Geometry: see drawing. Coordinates: mm, zero at the bounding-box minimum. A direction names the side the tool comes from. Coordinates: 2 decimals unless noted, no trailing zeros. Loops run counter-clockwise (first coordinate to the right, second up) from the corner with the lowest first, then second, coordinate; pieces in that order, holes last. Notation, with made-up numbers: (55, 51) -> (89, 51) arc R10 ccw to (89, 64) -> close; hole circle Ø11 at (6, -28). An arc over 180 degrees is marked (long way). One line per item, written item: value. Start each with the question number.
Item 1: Contact query for flat-ended pins moving along their axis: pin 1 Ø8 at (y, z) = (35.5, 21.5) entering from -X; pin 2 Ø1.5 at (x, z) = (17, 10) entering from +Y. Output: stop coordinate, or through.
Item 2: Ray query, probe 1 along X at (y, z) = (38, 68.5); probe 2 along Y at (x, z) = (50, 55.5). Return the intervals inside material, ascending. Write a range as from..to.
Item 3: Section query D-D on x = 21. Return loops of the section in (y, z), then the cut area to 3 significant figures.
Item 4: Section query A-A on y = 27. Return loops of the section in (x, z), then the cut area to 3 significant figures.
Item 5: Set-up query: the marked faces 1 and 2. Return all of +Z, -Z, +X, -X, +Y, -Y with unobstructed straight access to the full face (end or side cutting, diameter ignored); none if empty.
Item 6: Section query B-B on z = 39.5. Return loops of the section in (x, y), then the cut area to 3 significant figures.
Item 7: Section query C-C on z = 49.5. Return loops of the section in (x, y), then the cut area to 3 significant figures.
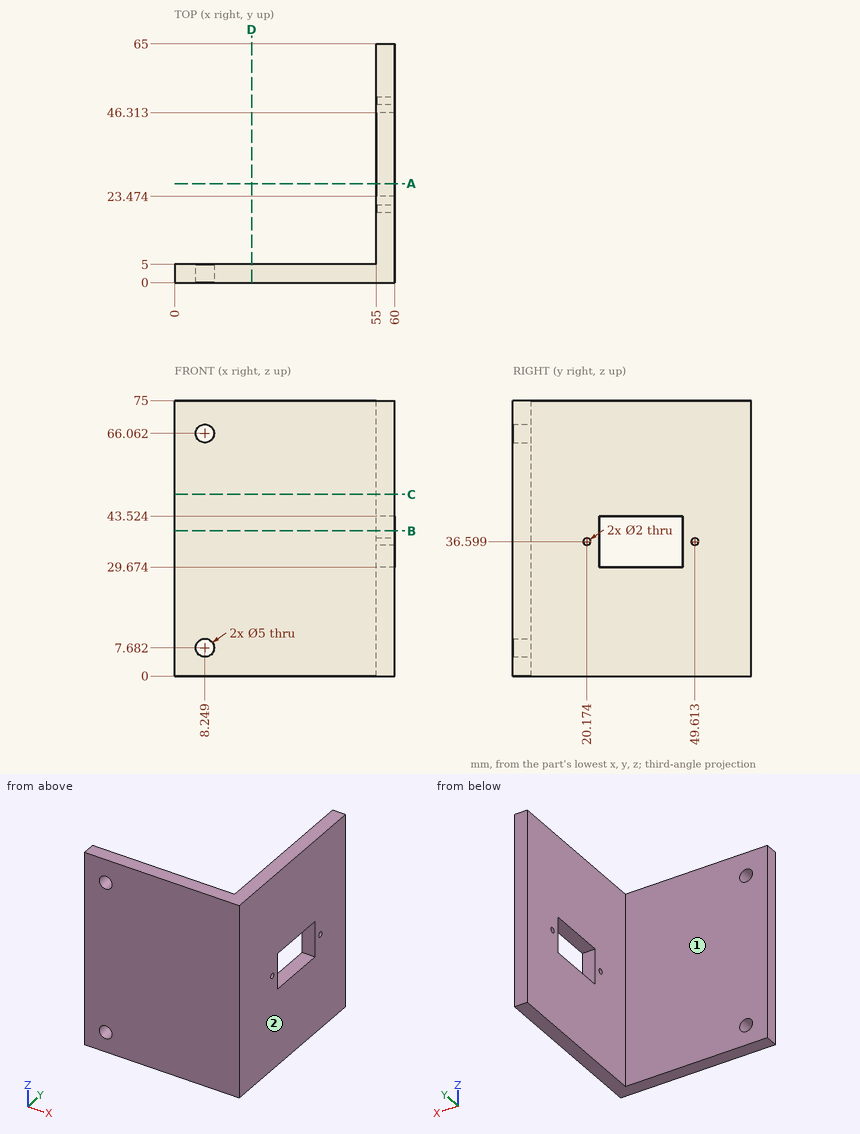
Reply:
1. pin 1: stops at x = 55
1. pin 2: stops at y = 5
2. probe 1: x = 55..60
2. probe 2: y = 0..5
3. outline: (0, 0) -> (5, 0) -> (5, 75) -> (0, 75) -> close
3. area: 375 mm²
4. outline: (55, 0) -> (60, 0) -> (60, 29.67) -> (55, 29.67) -> close; (55, 43.52) -> (60, 43.52) -> (60, 75) -> (55, 75) -> close
4. area: 306 mm²
5. face 1: +Z, -Z, -X, +Y
5. face 2: +Z, -Z, +X, +Y, -Y
6. outline: (0, 0) -> (60, 0) -> (60, 23.47) -> (55, 23.47) -> (55, 5) -> (0, 5) -> close; (55, 46.31) -> (60, 46.31) -> (60, 65) -> (55, 65) -> close
6. area: 486 mm²
7. outline: (0, 0) -> (60, 0) -> (60, 65) -> (55, 65) -> (55, 5) -> (0, 5) -> close
7. area: 600 mm²
